Input: part model. Units: mm. Frame: model coordinates. Give positions to 0.01 mm unless a question says otherwise; leave off trailing zeros. Order: outer loops, then holes, each group sorted by start corner. A loop starts at its lowest first (then second) coordinate and runs counter-clockwise, first axis right, second up. Notation, with made-up numbers: (-7.5, -8) - (26.5, -8) arc R28 ccw to (26.5, 18) - close; hole circle Ø4 at (88, -6.5). An arc over 180 degrees is marked (long way). Use a Markdown table: item, result.
from build123d import *

# Parameters (mm, degrees)
SKETCH1_W           = 60
SKETCH1_H           = 60
BOSS_EXTRUDE1_DEPTH = 1
SKETCH2_R           = 2
CUT_EXTRUDE1_DEPTH  = 2
SKETCH4_R           = 15.875
CUT_EXTRUDE3_DEPTH  = 10


with BuildPart() as part:
    # Sketch1 → Boss-Extrude1 (new body)
    with BuildSketch(Plane(origin=(0, 0, 0), x_dir=(1, 0, 0), z_dir=(0, 1, 0))):
        Rectangle(SKETCH1_W, SKETCH1_H)
    extrude(amount=BOSS_EXTRUDE1_DEPTH)

    # Sketch2 → Cut-Extrude1 (cut, through all)
    with BuildSketch(Plane(origin=(0, 1, 0), x_dir=(1, 0, 0), z_dir=(0, 1, 0))):
        with Locations((-26, 26)):
            Circle(SKETCH2_R)
        with Locations((0, 26)):
            Circle(SKETCH2_R)
        with Locations((26, 26)):
            Circle(SKETCH2_R)
        with Locations((26, -26)):
            Circle(SKETCH2_R)
        with Locations((0, -26)):
            Circle(SKETCH2_R)
        with Locations((-26, -26)):
            Circle(SKETCH2_R)
    extrude(amount=-CUT_EXTRUDE1_DEPTH, mode=Mode.SUBTRACT)

    # Sketch4 → Cut-Extrude3 (cut)
    with BuildSketch(Plane(origin=(0, 1, 0), x_dir=(1, 0, 0), z_dir=(0, 1, 0))):
        Circle(SKETCH4_R)
    extrude(amount=-CUT_EXTRUDE3_DEPTH, mode=Mode.SUBTRACT)


solid = part.part
1. Section query D-D (z = 26). Return loops of the section in (x, y), then the cut area to 3 significant figures.
Response:
| item | result |
|---|---|
| outline | (-30, 0) - (-28, 0) - (-28, 1) - (-30, 1) - close; (-24, 0) - (-2, 0) - (-2, 1) - (-24, 1) - close; (2, 0) - (24, 0) - (24, 1) - (2, 1) - close; (28, 0) - (30, 0) - (30, 1) - (28, 1) - close |
| area | 48.0 mm^2 |
2. Section query B-B (z = 0). Return loops of the section in (x, y) (3 decimals).
Response:
| item | result |
|---|---|
| outline | (-30, 0) - (-15.875, 0) - (-15.875, 1) - (-30, 1) - close; (15.875, 0) - (30, 0) - (30, 1) - (15.875, 1) - close |
3. Material intervals for line 1 along Z through (x, y) = (-26, 0.6); line 2 along Z through (x, y) = (0, 0.7) (3 decimals); line 3 along X through (y, z) = (0.75, -26), sorted ascending.
Response:
| item | result |
|---|---|
| line 1 | z = -30 to -28, -24 to 24, 28 to 30 |
| line 2 | z = -30 to -28, -24 to -15.875, 15.875 to 24, 28 to 30 |
| line 3 | x = -30 to -28, -24 to -2, 2 to 24, 28 to 30 |
4. Section query C-C (y = 0.15). Return loops of the section in (x, z) (3 decimals), then the cut area to 3 significant figures.
Response:
| item | result |
|---|---|
| outline | (-30, -30) - (30, -30) - (30, 30) - (-30, 30) - close; hole circle Ø4 at (-26, -26); hole circle Ø4 at (-26, 26); hole circle Ø31.75 at (0, 0); hole circle Ø4 at (0, -26); hole circle Ø4 at (0, 26); hole circle Ø4 at (26, -26); hole circle Ø4 at (26, 26) |
| area | 2,730 mm^2 |
5. Section query A-A (x = 0). Return loops of the section in (y, z) (3 decimals), then the cut area to 4 significant figures.
Response:
| item | result |
|---|---|
| outline | (0, -30) - (1, -30) - (1, -28) - (0, -28) - close; (0, -24) - (1, -24) - (1, -15.875) - (0, -15.875) - close; (0, 15.875) - (1, 15.875) - (1, 24) - (0, 24) - close; (0, 28) - (1, 28) - (1, 30) - (0, 30) - close |
| area | 20.25 mm^2 |
6. Mould query, pull axis Z, two halves, no side actions, for faces 1 (the face through (-26.434, 0.507, 27.952)), 2 (the face through (-14, 1, -14)). Classes: pulls with the +Z half, pulls with the -Z half, needs draft (parallel to the pull), parting line crosses it, or undercut.
Response:
| item | result |
|---|---|
| face 1 | undercut |
| face 2 | needs draft |
